Could you check a few things on this model? Use its own coordinates, in mm. A direction names the side the tool comes from. Give positions to 0.01 mm unless a question says otherwise; leave off trailing zeros. Loops run counter-clockwise (first coordinate to the right, second up) from the corner with the lowest first, then second, coordinate; pieces in that order, holes last. Notation, with made-up numbers: M 63,-13 L 116,-13 A18 ccw 116,2 Z; hole C -27,1.25 d11. An arc over 180 degrees is marked long. Use a Markdown table: item, result. Add a question column.
1) Which directions (+Z, -Z, +X, -X, +Y, -Y) give clear straight access to the entire face, cutting with the end or side of a thin tool? Please do faces 4 (the cylindrical face through (-93.62, 174.09, 647.06)), 5 (the flat face through (50.017, 4, 461)).
2) If I drill on line 1 along Y through (x, z) = (95, 285.5); line 2 along X through (y, z) = (172, 413); line 3 along Y through (x, z) = (-96, 594), over which ranges is the centre line in solid material (lowest first)? Write a range as [from, to].
3) Suppose I cut it at A-A on z = 457.2. List the corners of the cut face in (x, y) for me.
4) Suppose I cut it at D-D on x = 27. List the corners of the cut face in (y, z) for me, and give its area (3 significant figures).
5) Suppose I cut it at C-C on x = 118. List the corners of the cut face in (y, z) for me, and give its area (3 significant figures).
6) We'd pull the mould along Y, two halves only. Please class faces 1 (the conical face through (136.8, 11.3, 715)), 2 (the conical face through (148.104, 12.069, 731.429)), 3 (the flat face through (-50.017, 4, 454)): +Y half, -Y half, draft (parallel to the pull), parting line (faces both ways), or undercut.
7) Suppose I cut it at B-B on y = 0. List the corners of the cut face in (x, z) for me, and give its area (3 significant figures).
8) Will these pins go through, and if not, where does the flat tip stop? pin 1 Ø8 at (x, z) = (6, 770) entering from -Y; pin 2 Ø5 at (x, z) = (-47.5, 123.5) entering from -Y; pin 3 Ø4 at (x, y) = (-74, 232) entering from -Z.
```python
from build123d import *


with BuildPart() as f1:
    # F0 (on Front) → F1 (revolve)
    with BuildSketch(Plane.XZ):
        with BuildLine():
            ThreePointArc((-63.928831, 36.909328), (-36.909328, 9.889825), (0, 0))
            ThreePointArc((0, 0), (36.909328, 9.889825), (63.928831, 36.909328))
            Line((63.928831, 36.909328), (152.4, 190.145887))
            Line((152.4, 190.145887), (136.012062, 199.607468))
            Line((136.012062, 199.607468), (50.016642, 199.607468))
            Line((50.016642, 199.607468), (50.016642, 457.2))
            Line((50.016642, 457.2), (0, 457.2))
            Line((0, 457.2), (-50.016642, 457.2))
            Line((-50.016642, 457.2), (-50.016642, 199.607468))
            Line((-50.016642, 199.607468), (-136.012062, 199.607468))
            Line((-136.012062, 199.607468), (-152.4, 190.145887))
            Line((-152.4, 190.145887), (-63.928831, 36.909328))
        make_face()
    revolve(axis=Axis((25.008321, 0, 457.2), (1, 0, 0)))


solid = f1.part
```
Answer block:
| question | item | result |
|---|---|---|
| 1 | face 4 | -X |
| 1 | face 5 | +X |
| 2 | line 1 | y = [-323.76, -192.02], [192.02, 323.76] |
| 2 | line 2 | x = [-50.02, 50.02] |
| 2 | line 3 | y = [-338.12, -218.27], [218.27, 338.12] |
| 3 | outline | M -152.4,-267.05 L -63.93,-420.29 A73.82 ccw 0,-457.2 A73.82 ccw 63.93,-420.29 L 152.4,-267.05 L 136.01,-257.59 L 50.02,-257.59 L 50.02,257.59 L 136.01,257.59 L 152.4,267.05 L 63.93,420.29 A73.82 ccw 0,457.2 A73.82 ccw -63.93,420.29 L -152.4,267.05 L -136.01,257.59 L -50.02,257.59 L -50.02,-257.59 L -136.01,-257.59 Z |
| 4 | outline | C 0,457.2 d904.17 |
| 4 | area | 642,000 mm^2 |
| 5 | outline | C 0,457.2 d653.27; hole C 0,457.2 d515.19 |
| 5 | area | 127,000 mm^2 |
| 6 | face 1 | undercut |
| 6 | face 2 | parting line |
| 6 | face 3 | undercut |
| 7 | outline | M -152.4,190.15 L -63.93,36.91 A73.82 ccw 0,0 A73.82 ccw 63.93,36.91 L 152.4,190.15 L 136.01,199.61 L 50.02,199.61 L 50.02,714.79 L 136.01,714.79 L 152.4,724.25 L 63.93,877.49 A73.82 ccw 0,914.4 A73.82 ccw -63.93,877.49 L -152.4,724.25 L -136.01,714.79 L -50.02,714.79 L -50.02,199.61 L -136.01,199.61 Z |
| 7 | area | 130,000 mm^2 |
| 8 | pin 1 | stops at y = -336.85 |
| 8 | pin 2 | stops at y = -290.85 |
| 8 | pin 3 | stops at z = 123.41 |
